from build123d import *

# Parameters (mm, degrees)
SKETCH_1_R          = 3.2
SKETCH_1_R_2        = 1.8
SKETCH_1_R_3        = 5.7
SKETCH_1_R_4        = 1.7
EXTRUDE_1_DEPTH     = 3
SKETCH_2_R          = 10.5
EXTRUDE_2_DEPTH     = 7
SKETCH_4_R          = 1.7
CUT_EXTRUDE_1_DEPTH = 7
CUT_EXTRUDE_2_DEPTH = 3.5
SKETCH_6_R          = 5.7
CUT_EXTRUDE_3_DEPTH = 20
SKETCH_7_R          = 5
SKETCH_7_R_2        = 1.525
EXTRUDE_3_DEPTH     = 15
SKETCH_8_W          = 10
SKETCH_8_H          = 4
SKETCH_8_W_2        = 4
SKETCH_8_H_2        = 6
EXTRUDE_4_DEPTH     = 15
CUT_EXTRUDE_4_DEPTH = 15
CUT_EXTRUDE_5_DEPTH = 15
CUT_EXTRUDE_6_DEPTH = 15
SKETCH_12_W         = 25.575378798
SKETCH_12_H         = 2.842045507
EXTRUDE_5_DEPTH     = 7


with BuildPart() as part:
    # 草图1 → 凸台-拉伸1 (new body)
    with BuildSketch(Plane(origin=(0, 0, 0), x_dir=(1, 0, 0), z_dir=(0, 1, 0))):
        with BuildLine():
            Line((-35.081832586, -10), (-40, -10))
            Line((-40, -10), (-40, 10))
            Line((-40, 10), (-11.180339887, 10))
            ThreePointArc((-11.180339887, 10), (0, 15), (11.180339887, 10))
            Line((11.180339887, 10), (40, 10))
            Line((40, 10), (40, -10))
            Line((40, -10), (20, -10))
            Line((20, -10), (38.795982487, -42.134997854))
            Line((38.795982487, -42.134997854), (23.493176713, -51.085714784))
            Line((23.493176713, -51.085714784), (10.00055485, -20.000324527))
            Line((10.00055485, -20.000324527), (-9.99944515, -20.000324527))
            Line((-9.99944515, -20.000324527), (-23.493239928, -51.085714784))
            Line((-23.493239928, -51.085714784), (-38.79573581, -42.1354119))
            Line((-38.79573581, -42.1354119), (-20, -10))
            Line((-20, -10), (-35.081832586, -10))
        make_face()
        with Locations(Location((35, 0, 0), (0, 0, 270))):
            Circle(SKETCH_1_R, mode=Mode.SUBTRACT)
        with Locations(Location((-15.5, -15.5, 0), (0, 0, 270))):
            Circle(SKETCH_1_R_2, mode=Mode.SUBTRACT)
        with Locations(Location((15.5, -15.5, 0), (0, 0, 270))):
            Circle(SKETCH_1_R_2, mode=Mode.SUBTRACT)
        with Locations(Location((-35, 0, 0), (0, 0, 270))):
            Circle(SKETCH_1_R, mode=Mode.SUBTRACT)
        with Locations(Location((0, 0, 0), (0, 0, 270))):
            Circle(SKETCH_1_R_3, mode=Mode.SUBTRACT)
        with Locations(Location((-8, 0, 0), (0, 0, 270))):
            Circle(SKETCH_1_R_4, mode=Mode.SUBTRACT)
        with Locations(Location((0, 8, 0), (0, 0, 270))):
            Circle(SKETCH_1_R_4, mode=Mode.SUBTRACT)
        with Locations(Location((8, 0, 0), (0, 0, 270))):
            Circle(SKETCH_1_R_4, mode=Mode.SUBTRACT)
        with Locations(Location((0, -8, 0), (0, 0, 270))):
            Circle(SKETCH_1_R_4, mode=Mode.SUBTRACT)
        with BuildLine():
            Line((-16.131862345, -20.121977189), (-28.419219954, -44.445930008))
            ThreePointArc((-28.419219954, -44.445930008), (-30.461319047, -45.117305053), (-31.132694091, -43.07520596))
            Line((-31.132694091, -43.07520596), (-18.845336482, -18.75125314))
            ThreePointArc((-18.845336482, -18.75125314), (-16.803237389, -18.079878096), (-16.131862345, -20.121977189))
        make_face(mode=Mode.SUBTRACT)
        with BuildLine():
            Line((19.251434516, -19.436615165), (31.203359651, -43.037711333))
            ThreePointArc((31.203359651, -43.037711333), (30.498813674, -45.187970612), (28.348554395, -44.483424635))
            Line((28.348554395, -44.483424635), (16.39662926, -20.882328467))
            ThreePointArc((16.39662926, -20.882328467), (17.101175237, -18.732069188), (19.251434516, -19.436615165))
        make_face(mode=Mode.SUBTRACT)
    extrude(amount=EXTRUDE_1_DEPTH)

    # 草图2 → 凸台-拉伸2 (add)
    with BuildSketch(Plane(origin=(0, 3, 0), x_dir=(1, 0, 0), z_dir=(0, 1, 0))):
        with Locations(Location((0, 0, 0), (0, 0, 270))):
            Circle(SKETCH_2_R)
    extrude(amount=EXTRUDE_2_DEPTH)

    # 草图4 → 切除-拉伸1 (cut)
    with BuildSketch(Plane.XZ.offset(-3)):
        with Locations(Location((0, -8, 0), (0, 0, 270))):
            Circle(SKETCH_4_R)
        with Locations(Location((-8, 0, 0), (0, 0, 270))):
            Circle(SKETCH_4_R)
        with Locations(Location((8, 0, 0), (0, 0, 270))):
            Circle(SKETCH_4_R)
        with Locations(Location((0, 8, 0), (0, 0, 270))):
            Circle(SKETCH_4_R)
    extrude(amount=-CUT_EXTRUDE_1_DEPTH, mode=Mode.SUBTRACT)

    # 草图5 → 切除-拉伸2 (cut)
    with BuildSketch(Plane(origin=(0, 3, 0), x_dir=(1, 0, 0), z_dir=(0, 1, 0))):
        Polygon((-4.766838493, 0), (-6.383419246, 2.8), (-11.233161507, 2.8), (-11.233161507, -2.8), (-6.383419246, -2.8), align=None)
        Polygon((4.766838493, 0), (6.383419246, -2.8), (11.233161507, -2.8), (11.233161507, 2.8), (6.383419246, 2.8), align=None)
        Polygon((-2.8, 11.233161507), (-2.8, 6.383419246), (0, 4.766838493), (2.8, 6.383419246), (2.8, 11.233161507), align=None)
        Polygon((0, -4.766838493), (-2.8, -6.383419246), (-2.8, -11.233161507), (2.8, -11.233161507), (2.8, -6.383419246), align=None)
    extrude(amount=CUT_EXTRUDE_2_DEPTH, mode=Mode.SUBTRACT)

    # 草图6 → 切除-拉伸3 (cut)
    with BuildSketch(Plane.XZ.offset(-3)):
        with Locations(Location((0, 0, 0), (0, 0, 90))):
            Circle(SKETCH_6_R)
    extrude(amount=-CUT_EXTRUDE_3_DEPTH, mode=Mode.SUBTRACT)

    # 草图7 → 凸台-拉伸3 (add)
    # profile 1 of 2: a face of its own
    with BuildSketch(Plane(origin=(0, 3, 0), x_dir=(1, 0, 0), z_dir=(0, 1, 0))):
        with Locations(Location((-35, 0, 0), (0, 0, 180))):
            Circle(SKETCH_7_R)
        with Locations(Location((-35, 0, 0), (0, 0, 270))):
            Circle(SKETCH_7_R_2, mode=Mode.SUBTRACT)
    # profile 2 of 2: a face of its own
    with BuildSketch(Plane(origin=(0, 3, 0), x_dir=(1, 0, 0), z_dir=(0, 1, 0))):
        with Locations((35, 0)):
            Circle(SKETCH_7_R)
        with Locations(Location((35, 0, 0), (0, 0, 270))):
            Circle(SKETCH_7_R_2, mode=Mode.SUBTRACT)
    extrude(amount=EXTRUDE_3_DEPTH)

    # 草图8 → 凸台-拉伸4 (add)
    with BuildSketch(Plane(origin=(0, 3, 0), x_dir=(1, 0, 0), z_dir=(0, 1, 0))):
        with Locations((-26, 0)):
            Rectangle(SKETCH_8_W, SKETCH_8_H)
        with Locations((-35, 7)):
            Rectangle(SKETCH_8_W_2, SKETCH_8_H_2)
        with Locations((-35, -7)):
            Rectangle(SKETCH_8_W_2, SKETCH_8_H_2)
        with Locations((26, 0)):
            Rectangle(SKETCH_8_W, SKETCH_8_H)
        with Locations((35, 7)):
            Rectangle(SKETCH_8_W_2, SKETCH_8_H_2)
        with Locations((35, -7)):
            Rectangle(SKETCH_8_W_2, SKETCH_8_H_2)
    extrude(amount=EXTRUDE_4_DEPTH)

    # 草图9 → 切除-拉伸4 (cut)
    with BuildSketch(Plane.XY.offset(2)):
        Polygon((-30.417424305, 18), (-21, 3), (-21, 18), align=None)
        Polygon((21, 3), (30.417424305, 18), (21, 18), align=None)
    extrude(amount=-CUT_EXTRUDE_4_DEPTH, mode=Mode.SUBTRACT)

    # 草图10 → 切除-拉伸5 (cut)
    with BuildSketch(Plane.ZY.offset(-33)):
        Polygon((-4.582575695, 18), (-10, 3), (-10, 18), align=None)
        Polygon((4.582575695, 18), (10, 18), (10, 3), align=None)
    extrude(amount=-CUT_EXTRUDE_5_DEPTH, mode=Mode.SUBTRACT)

    # 草图11 → 切除-拉伸6 (cut)
    with BuildSketch(Plane(origin=(-33, 0, 0), x_dir=(0, 0, -1), z_dir=(1, 0, 0))):
        Polygon((-4.582575695, 18), (-10, 3), (-10, 18), align=None)
        Polygon((4.582575695, 18), (10, 3), (10, 18), align=None)
    extrude(amount=-CUT_EXTRUDE_6_DEPTH, mode=Mode.SUBTRACT)

    # 草图12 → 凸台-拉伸5 (add)
    with BuildSketch(Plane(origin=(0, 3, 0), x_dir=(1, 0, 0), z_dir=(0, 1, 0))):
        with Locations((-20.212310601, -6.003598449)):
            Rectangle(SKETCH_12_W, SKETCH_12_H)
        with Locations((-20.212310601, 6.003598449)):
            Rectangle(SKETCH_12_W, SKETCH_12_H)
        with Locations((20.212310601, 6.003598449)):
            Rectangle(SKETCH_12_W, SKETCH_12_H)
        with Locations((20.212310601, -6.003598449)):
            Rectangle(SKETCH_12_W, SKETCH_12_H)
    extrude(amount=EXTRUDE_5_DEPTH)


solid = part.part
Part model, mm, in its own coordinate system. A direction names the side the tool comes from. Coordinates: 2 decimals unless noted, no trailing zeros. Order: outer loops, then holes, each group sorted by start corner. A loop starts at its lowest first (then second) coordinate and runs counter-clockwise, first axis right, second up.
(1) Pin check, flat tips, straight feed: pin 1 Ø5 at (x, z) = (-18, -4.5) entering from +Y; pin 2 Ø6 at (y, z) = (11, -5) entering from -X; pin 3 Ø7.5 at (x, y) = (-25, 13.5) entering from +Z. Stop position of each tip, or through.
Check sheet entries:
pin 1: stops at y = 10
pin 2: stops at x = -39.58
pin 3: stops at z = 7.42
(2) Tool access for faces 4 (the face through (0.1, 7.2, -10.5)), 5 (the face through (-31.827, 1.479, -0.417)), 6 (the face through (22.456, 1.479, 32.848)), 7 (the face through (-20, 6, 7.425)), 8 (the face through (10, 6.5, -1)): list every direction of +Z, -Z, +X, -X, +Y, -Y with a clear straight run to the whole face (end or side of a thin tool).
Check sheet entries:
face 4: -Z, +Y
face 5: -Y
face 6: +Y, -Y
face 7: +Z, +Y
face 8: none
(3) Probe L1, parallel to Z at x = -29, y = 7; L2, parallel to X at y = 1.15, z = -8; L3, parallel to X at y = 1.1, z = 0. List the from-to ranges inside material, lowest first.
Check sheet entries:
L1: z = -7.42 to -4.58, -2 to 2, 4.58 to 7.42
L2: x = -40 to -1.7, 1.7 to 40
L3: x = -40 to -38.2, -31.8 to -9.7, -6.3 to -5.7, 5.7 to 6.3, 9.7 to 31.8, 38.2 to 40
(4) Slice it at A-A, the plane x = 25. Write the cut outline in (y, z), and give its area (3 significant figures).
Check sheet entries:
outline: (0, -10) - (3, -10) - (3, -7.42) - (10, -7.42) - (10, -4.58) - (3, -4.58) - (3, -2) - (9.37, -2) - (9.37, 2) - (3, 2) - (3, 4.58) - (10, 4.58) - (10, 7.42) - (3, 7.42) - (3, 10) - (0, 10) - close; (0, 18.55) - (3, 18.55) - (3, 30.79) - (0, 30.79) - close; (0, 37.87) - (3, 37.87) - (3, 50.2) - (0, 50.2) - close
area: 199 mm2
(5) Pull direction Y, two halves, no side cores. Call faces 1 (the face through (34.972, 10.395, 7.329)), 2 (the face through (-30.431, 1.479, 45.132)), 3 (the face through (0, 6.5, -10)): pulls with the +Y half, pulls with the -Y half, needs draft (parallel to the pull), parting line crosses it, or undercut.
Check sheet entries:
face 1: pulls with the +Y half
face 2: needs draft
face 3: undercut
(6) Slice it at C-C, the plane z = 15.5. Write the cut outline in (x, y).
Check sheet entries:
outline: (-23.22, 0) - (-17.3, 0) - (-17.3, 3) - (-23.22, 3) - close; (-13.7, 0) - (13.7, 0) - (13.7, 3) - (-13.7, 3) - close; (17.3, 0) - (23.22, 0) - (23.22, 3) - (17.3, 3) - close
(7) Slice it at D-D, the plane y = 5.5. State how many separate pieces and enclosed holes the cut face has, and give its area (3 significant figures).
Check sheet entries:
separate pieces: 2
enclosed holes: 2
area: 691 mm2
(8) Slice it at B-B, the plane z = -8.5. Write the cut outline in (x, y), and give its area (3 significant figures).
Check sheet entries:
outline: (-40, 0) - (-1.62, 0) - (-1.62, 3) - (-2.8, 3) - (-2.8, 6.5) - (-1.62, 6.5) - (-1.62, 10) - (-6.16, 10) - (-6.16, 3) - (-33, 3) - (-33, 7.15) - (-37, 7.15) - (-37, 3) - (-40, 3) - close; (1.62, 0) - (40, 0) - (40, 3) - (37, 3) - (37, 7.15) - (33, 7.15) - (33, 3) - (6.16, 3) - (6.16, 10) - (1.62, 10) - (1.62, 6.5) - (2.8, 6.5) - (2.8, 3) - (1.62, 3) - close
area: 319 mm2
